Design review of the part shown in the three views and the two pictorial views. Dimensions are in mm from the part's minimum x, y and z. A direction names the side the tool comes from. Coordinates: 2 decimals unless noted, no trailing zeros. Order: outer loops, then holes, each group sorted by start corner. A loop starts at its lowest first (then second) coordinate and runs counter-clockwise, first axis right, second up. Notation, with made-up numbers: (-9.75, 6.25) -> (3.25, 6.25) arc R26 cw to (3.25, 44.25) -> close; hole circle Ø7 at (70.5, 69). An arc over 180 degrees is marked (long way). Write item = value, one per line. Start each with the question number.
1) Consider section B-B on x = 6. Give the boundary of the cut face in (y, z), and give its area (3 significant figures).
2) Consider section C-C on y = 37.25. Give the boundary of the cut face in (x, z).
3) Consider section A-A on y = 69.5. Give the boundary of the cut face in (x, z), and give its area (4 significant figures).
4) Wall thickness on probe 1 along X at (y, z) = (5, 46); probe 2 along Y at (x, z) = (19.85, 30); probe 3 along Y at (x, z) = (33.7, 46.7): over which ranges is each line inside the solid? List them lowest first. Write a range as [from, to].
5) Consider section D-D on z = 22. Give the boundary of the cut face in (x, y).
6) Draft analysis for pull direction Y (two halves, no side actions). For the marked faces 1, 2, 3 and 4, state which applies: +Y half, -Y half, draft (parallel to the pull), parting line (faces both ways), or undercut.
7) Insertion check: pin 1 Ø20 at (x, z) = (19.5, 12) entering from -Y; pin 2 Ø15 at (x, z) = (19.5, 18) entering from +Y; pin 3 Ø4 at (x, y) = (25, 5) entering from -Z. Each pin has a flat end and moves straight along its axis. Give the tip position at first contact, or say it passes through.
8) Machinability: for the marked faces 5, 6 and 7, which of the approach directions +Z, -Z, +X, -X, +Y, -Y give a long, thin tool a straight path to every point of the face, cutting with its end or side? Answer none if there is none.
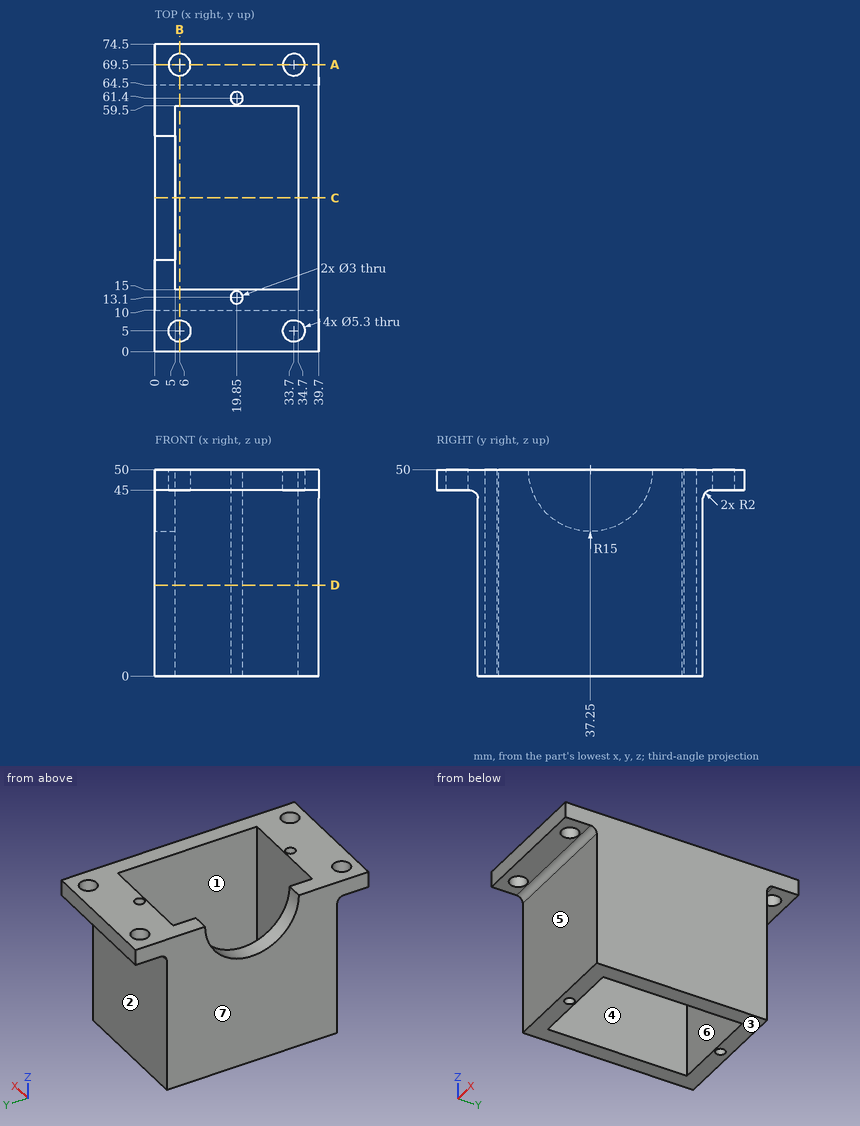
Answer sheet:
q1.outline = (0, 45) -> (2.35, 45) -> (2.35, 50) -> (0, 50) -> close; (7.65, 45) -> (8, 45) arc R2 cw to (10, 43) -> (10, 0) -> (15, 0) -> (15, 50) -> (7.65, 50) -> close; (59.5, 0) -> (64.5, 0) -> (64.5, 43) arc R2 cw to (66.5, 45) -> (66.85, 45) -> (66.85, 50) -> (59.5, 50) -> close; (72.15, 45) -> (74.5, 45) -> (74.5, 50) -> (72.15, 50) -> close
q1.area = 549 mm2
q2.outline = (0, 0) -> (5, 0) -> (5, 35) -> (0, 35) -> close; (34.7, 0) -> (39.7, 0) -> (39.7, 50) -> (34.7, 50) -> close
q3.outline = (0, 45) -> (3.35, 45) -> (3.35, 50) -> (0, 50) -> close; (8.65, 45) -> (31.05, 45) -> (31.05, 50) -> (8.65, 50) -> close; (36.35, 45) -> (39.7, 45) -> (39.7, 50) -> (36.35, 50) -> close
q3.area = 145.5 mm2
q4.probe_1 = [0, 3.35], [8.65, 31.05], [36.35, 39.7]
q4.probe_2 = [10, 11.6], [14.6, 15], [59.5, 59.9], [62.9, 64.5]
q4.probe_3 = [0, 2.35], [7.65, 15], [59.5, 66.85], [72.15, 74.5]
q5.outline = (0, 10) -> (39.7, 10) -> (39.7, 64.5) -> (0, 64.5) -> close; hole (5, 15) -> (34.7, 15) -> (34.7, 59.5) -> (5, 59.5) -> close; hole circle Ø3 at (19.85, 13.1); hole circle Ø3 at (19.85, 61.4)
q6.face_1 = undercut
q6.face_2 = +Y half
q6.face_3 = draft
q6.face_4 = undercut
q7.pin_1 = 10
q7.pin_2 = 64.5
q7.pin_3 = 45
q8.face_5 = -Z, +X, -X, -Y
q8.face_6 = +Z, -Z
q8.face_7 = +Z, -Z, -X, +Y, -Y
